Design review of the part built by this model. Coordinates are the model's own, in mm. Give positions to 0.01 mm unless a question says otherwise; leave off trailing zeros. Loops run counter-clockwise (first coordinate to the right, second up) from the corner with the lowest first, then second, coordinate; pieces in that order, holes last. Notation, with made-up numbers: M 58,65.25 L 99,65.25 A22 ccw 99,87.25 Z; hole C -40,27.5 d8. An arc over 180 degrees is marked long. Answer as CSV lines item,"result".
Autodesk Fusion 360 part; units mm, degrees
sketch "Sketch1" plane through (0, 0, 0) normal (0, 0, 1) x (1, 0, 0)
  line L0 (-81, 18) -> (81, 18)
  line L1 (88, 11) -> (88, -11)
  line L2 (81, -18) -> (-81, -18)
  line L3 (-88, -11) -> (-88, 11)
  line L4 (-88, 18) -> (88, -18) construction
  line L5 (88, 18) -> (-88, -18) construction
  arc A0 (-81, 18) -> (-88, 11) centre (-81, 11) ccw
  arc A1 (-88, -11) -> (-81, -18) centre (-81, -11) ccw
  arc A2 (81, -18) -> (88, -11) centre (81, -11) ccw
  arc A3 (88, 11) -> (81, 18) centre (81, 11) ccw
  line L6 (0, 0) -> (27, 0) construction
  circle A4 centre (-84, 0) radius 1.5
  line L7 (0, 0) -> (0, 18) construction
  circle A5 centre (84, 0) radius 1.5
  dimension "d28" = 176
  dimension "d29" = 36
  dimension "d30" = 7
  dimension "d35" = 3
  dimension "d36" = 4
  dimension "d37" = 18
extrude "Extrude7" add sketch "Sketch1" along normal blind 3
sketch "Sketch3" plane through (0, 0, 3) normal (0, 0, 1) x (-1, 0, 0)
  circle A0 centre (0, -13) radius 1.5
  circle A1 centre (-85, 0) radius 1.5
  circle A2 centre (0, 13) radius 1.5
  circle A3 centre (85, 0) radius 1.5
  line L0 (-79, 9) -> (79, 9)
  line L1 (79, 9) -> (79, -9)
  line L2 (79, -9) -> (-79, -9)
  line L3 (-79, -9) -> (-79, 9)
  arc A4 (-83, 18) -> (-90, 11) centre (-83, 11) ccw
  line L4 (-90, 11) -> (-90, -11)
  arc A5 (-90, -11) -> (-83, -18) centre (-83, -11) ccw
  line L5 (-83, -18) -> (83, -18)
  arc A6 (83, -18) -> (90, -11) centre (83, -11) ccw
  line L6 (90, -11) -> (90, 11)
  arc A7 (90, 11) -> (83, 18) centre (83, 11) ccw
  line L7 (83, 18) -> (-83, 18)
  circle A8 centre (0, 13) radius 1.5
1. We need section B-B, the plane x = 84. Write out the cut boundary in (y, z), plus the area to 3 significant figures.
Answer block:
outline,"M -17.32,0 L -1.5,0 L -1.5,3 L -17.32,3 Z; M 1.5,0 L 17.32,0 L 17.32,3 L 1.5,3 Z"
area,"94.9 mm²"
2. The part is to be moulded in two halves that separate along X. For faces 1 (the cylindrical face through (-82.57, -0.45, 1.48)), 2 (the cylindrical face through (85.9, 16, 1.5)), 3 (the flat face through (-1, 0, 3)), say which applies: pulls with the +X half, pulls with the -X half, needs draft (parallel to the pull), parting line crosses it, or undercut.
Answer block:
face 1,"undercut"
face 2,"pulls with the +X half"
face 3,"needs draft"
3. We need section A-A, the plane y = 0. Write out the cut boundary in (x, z).
Answer block:
outline,"M -88,0 L -85.5,0 L -85.5,3 L -88,3 Z; M -82.5,0 L 82.5,0 L 82.5,3 L -82.5,3 Z; M 85.5,0 L 88,0 L 88,3 L 85.5,3 Z"
4. For P1, Ø1.8, axis at x = -84, y = 0, coming from the -Z side; P2, Ø8, axis at x = -50.5, y = 12, coming from the -Z side, all flat-tipped, find the tip position at first contact; note any pin that passes through.
Answer block:
P1,"through"
P2,"z = 0"
5. To check wall thickness, follow L1, parallel to Y at x = -84, z = 0.9; L2, parallel to X at y = 15, z = 2.7; L3, parallel to X at y = -12, z = 2.5. State the ranges of each line that lie inside material, in increasing order. Write a range as [from, to].
Answer block:
L1,"[-17.32, -1.5], [1.5, 17.32]"
L2,"[-86.74, 86.74]"
L3,"[-87.93, 87.93]"
